For this review, take the finished solid that the model builds, in its own axes (mm). A direction names the side the tool comes from. Coordinates: 2 decimals unless noted, no trailing zeros. Order: outer loops, then holes, each group sorted by start corner. A loop starts at its lowest first (then second) coordinate and runs counter-clockwise, first axis right, second up.
from build123d import *

# Parameters (mm, degrees)
BASE_FLANGE1_DEPTH = 35
SKETCH3_R          = 5
SKETCH3_R_2        = 1.75
CUT_EXTRUDE1_DEPTH = 10
CHAMFER1_SIZE      = 5
SKETCH4_R          = 2.25
CUT_EXTRUDE2_DEPTH = 10


# Sheet-metal steps are written as plain solids
with BuildPart() as part:
    # Sketch1 → Base-Flange1 (new body)
    with BuildSketch(Plane.XY):
        with BuildLine():
            Line((-36, 0), (-4, 0))
            ThreePointArc((-4, 0), (-1.171572875, 1.171572875), (0, 4))
            Line((0, 4), (0, 45.5))
            Line((0, 45.5), (-2, 45.5))
            Line((-2, 45.5), (-2, 4))
            ThreePointArc((-2, 4), (-2.585786438, 2.585786438), (-4, 2))
            Line((-4, 2), (-36, 2))
            Line((-36, 2), (-36, 0))
        make_face()
    extrude(amount=BASE_FLANGE1_DEPTH)

    # Sketch3 → Cut-Extrude1 (cut)
    with BuildSketch(Plane(origin=(0, 0, 0), x_dir=(0, 0, -1), z_dir=(1, 0, 0))):
        with Locations((-17.5, 29)):
            Circle(SKETCH3_R)
        with Locations((-18.25, 11)):
            Circle(SKETCH3_R_2)
        with Locations((-18.25, 36.5)):
            Circle(SKETCH3_R_2)
    extrude(amount=-CUT_EXTRUDE1_DEPTH, mode=Mode.SUBTRACT)

    # Chamfer1
    chamfer1_edges = [part.edges().sort_by_distance(p)[0] for p in [
        (-1, 45.5, 35),
        (-36, 1, 35),
        (-1, 45.5, 0),
        (-36, 1, 0),
    ]]
    chamfer(chamfer1_edges, length=CHAMFER1_SIZE)

    # Sketch4 → Cut-Extrude2 (cut)
    with BuildSketch(Plane.XZ):
        with Locations((-28, 17.5)):
            Circle(SKETCH4_R)
        with Locations((-12, 17.5)):
            Circle(SKETCH4_R)
    extrude(amount=-CUT_EXTRUDE2_DEPTH, mode=Mode.SUBTRACT)


solid = part.part
1. Machinability: for faces 4 (the face through (0, 24, 21)), 5 (the face through (-2, 25, 21)), which of the approach directions +Z, -Z, +X, -X, +Y, -Y give a long, thin tool a straight path to every point of the face, cutting with its end or side? Answer none if there is none.
Answer below:
face 4: +Z, -Z, +X, +Y, -Y
face 5: +Z, -Z, -X, +Y
2. Clearance check with flat-ended pins moving along their axes: pin 1 Ø10 at (x, z) = (-26.5, 15) entering from +Y; pin 2 Ø10 at (y, z) = (11, 31) entering from -X. State where each tip first meets the part, or that it passes through.
Answer below:
pin 1: stops at y = 2
pin 2: stops at x = -2
3. Take a section at B-B, the plane x = -28. Give the boundary of the cut face in (y, z).
Answer below:
outline: (0, 0) - (2, 0) - (2, 15.25) - (0, 15.25) - close; (0, 19.75) - (2, 19.75) - (2, 35) - (0, 35) - close
4. To check wall thickness, follow L1, parallel to Y at x = -1.2, z = 17.5; L2, parallel to Y at x = -22.5, z = 22; L3, parallel to Y at x = -0.65, z = 18.25. State the ranges of each line that lie inside material, in increasing order.
Answer below:
L1: y = 1.14 to 9.42, 12.58 to 24, 34 to 34.92, 38.08 to 45.5
L2: y = 0 to 2
L3: y = 1.81 to 9.25, 12.75 to 24.06, 33.94 to 34.75, 38.25 to 45.5
5. The part is to be moulded in two halves that separate along Y. For faces 1 (the face through (-0.99, 35.44, 19.64)), 2 (the face through (-20, 0, 17)), 3 (the face through (-33, 1, 33)), say which applies: +Y half, -Y half, draft (parallel to the pull), parting line (faces both ways), or undercut.
Answer below:
face 1: undercut
face 2: -Y half
face 3: draft
6. Take a section at D-D, the plane z = 17.5. Give the boundary of the cut face in (x, y), plus the area to 3 significant figures.
Answer below:
outline: (-36, 0) - (-30.25, 0) - (-30.25, 2) - (-36, 2) - close; (-25.75, 0) - (-14.25, 0) - (-14.25, 2) - (-25.75, 2) - close; (-9.75, 0) - (-4, 0) arc R4 ccw to (0, 4) - (0, 9.42) - (-2, 9.42) - (-2, 4) arc R2 cw to (-4, 2) - (-9.75, 2) - close; (-2, 12.58) - (0, 12.58) - (0, 24) - (-2, 24) - close; (-2, 34) - (0, 34) - (0, 34.92) - (-2, 34.92) - close; (-2, 38.08) - (0, 38.08) - (0, 45.5) - (-2, 45.5) - close
area: 106 mm2
7. Take a section at A-A, the plane y = 11. Give the boundary of the cut face in (x, z).
Answer below:
outline: (-2, 0) - (0, 0) - (0, 16.5) - (-2, 16.5) - close; (-2, 20) - (0, 20) - (0, 35) - (-2, 35) - close
8. Take a section at C-C, the plane z = 27.5. Give the boundary of the cut face in (x, y), plus the area to 3 significant figures.
Answer below:
outline: (-36, 0) - (-4, 0) arc R4 ccw to (0, 4) - (0, 45.5) - (-2, 45.5) - (-2, 4) arc R2 cw to (-4, 2) - (-36, 2) - close
area: 156 mm2
